```python
from build123d import *

# Parameters (mm, degrees)
PAD003_DEPTH         = 42
SKETCH008_W          = 60
SKETCH008_H          = 34
POCKET004_DEPTH      = 15.001
SKETCH009_R          = 1.45
POCKET005_DEPTH      = 8
POCKET006_DEPTH      = 42.001
POCKET008_DEPTH      = 21.001
POCKET008_DEPTH_BACK = 21.001
SKETCH013_R          = 1.75
PAD004_DEPTH         = 4.5
POCKET_DEPTH         = 25.501
PAD015_DEPTH         = 25


with BuildPart() as part:
    # Sketch006 → Pad003 (new body)
    with BuildSketch(Plane.XZ):
        with BuildLine():
            Line((-16, 21), (16, 21))
            ThreePointArc((21, 16), (19.5355339059, 19.5355339059), (16, 21))
            Line((21, 16), (21, -16))
            ThreePointArc((16, -21), (19.5355339059, -19.5355339059), (21, -16))
            Line((16, -21), (-16, -21))
            ThreePointArc((-21, -16), (-19.5355339059, -19.5355339059), (-16, -21))
            Line((-21, -16), (-21, 16))
            ThreePointArc((-16, 21), (-19.5355339059, 19.5355339059), (-21, 16))
        make_face()
    extrude(amount=PAD003_DEPTH)

    # Sketch008 (on DatumPlane) → Pocket004 (cut, through all)
    with BuildSketch(Plane.XY.offset(6)):
        with Locations((0, -17)):
            Rectangle(SKETCH008_W, SKETCH008_H)
    extrude(amount=POCKET004_DEPTH, mode=Mode.SUBTRACT)

    # Sketch009 (on DatumPlane) → Pocket005 (cut)
    with BuildSketch(Plane.XZ.offset(42)):
        with Locations((-16, 16)):
            Circle(SKETCH009_R)
        with Locations((16, 16)):
            Circle(SKETCH009_R)
        with Locations((-16, -16)):
            Circle(SKETCH009_R)
        with Locations((16, -16)):
            Circle(SKETCH009_R)
    extrude(amount=-POCKET005_DEPTH, mode=Mode.SUBTRACT)

    # Sketch010 (on DatumPlane) → Pocket006 (cut, through all)
    with BuildSketch(Plane.XZ.offset(42)):
        with BuildLine():
            Line((-18.9580398915, 15.5), (-18.9580398915, -15.5))
            ThreePointArc((-15.5, -18.9580398915), (-13.8786796564, -13.8786796564), (-18.9580398915, -15.5))
            Line((-15.5, -18.9580398915), (15.5, -18.9580398915))
            ThreePointArc((18.9580398915, -15.5), (13.8786796564, -13.8786796564), (15.5, -18.9580398915))
            Line((18.9580398915, -15.5), (18.9580398915, 15.5))
            ThreePointArc((15.5, 18.9580398915), (13.8786796564, 13.8786796564), (18.9580398915, 15.5))
            Line((-15.5, 18.9580398915), (15.5, 18.9580398915))
            ThreePointArc((-18.9580398915, 15.5), (-13.8786796564, 13.8786796564), (-15.5, 18.9580398915))
        make_face()
    extrude(amount=-POCKET006_DEPTH, mode=Mode.SUBTRACT)

    # Sketch012 → Pocket008 (cut, two sides)
    with BuildSketch(Plane.YZ) as pocket008_sk:
        with BuildLine():
            ThreePointArc((-2.5, 0), (-6, 3.5), (-9.5, 0))
            Line((-9.5, 0), (-9.5, -9))
            ThreePointArc((-9.5, -9), (-6, -12.5), (-2.5, -9))
            Line((-2.5, -9), (-2.5, 0))
        make_face()
        with BuildLine():
            ThreePointArc((-12.5, 0), (-16, 3.5), (-19.5, 0))
            Line((-19.5, 0), (-19.5, -9))
            ThreePointArc((-19.5, -9), (-16, -12.5), (-12.5, -9))
            Line((-12.5, -9), (-12.5, 0))
        make_face()
    extrude(amount=-POCKET008_DEPTH, mode=Mode.SUBTRACT)
    extrude(pocket008_sk.sketch, amount=POCKET008_DEPTH_BACK, mode=Mode.SUBTRACT)

    # Sketch013 → Pad004 (join)
    with BuildSketch(Plane.XZ):
        with BuildLine():
            ThreePointArc((22.5, 5.5), (24.9748737342, 11.4748737342), (19, 9))
            Line((19.0000000001, 9), (19.0000000001, 2.0000200959))
            ThreePointArc((22.5, 5.5), (20.0251333708, 4.4748808391), (19.0000000001, 2.0000200959))
        make_face()
        with Locations((22.5, 9)):
            Circle(SKETCH013_R, mode=Mode.SUBTRACT)
        with BuildLine():
            ThreePointArc((-22.5, -18.5), (-24.9748737342, -24.4748737342), (-19, -22))
            ThreePointArc((-18.0892857143, -19.6450903436), (-18.7643912143, -20.7375618827), (-19, -22))
            Line((-20.1450903436, -17.5892857143), (-18.0892857143, -19.6450903436))
            ThreePointArc((-22.5, -18.5), (-21.2375618827, -18.2643912143), (-20.1450903436, -17.5892857143))
        make_face()
        with Locations((-22.5, -22)):
            Circle(SKETCH013_R, mode=Mode.SUBTRACT)
        with BuildLine():
            ThreePointArc((19, -22), (24.9748737342, -24.4748737342), (22.5, -18.5))
            ThreePointArc((20.1450903436, -17.5892857143), (21.2375618827, -18.2643912143), (22.5, -18.5))
            Line((18.0892857143, -19.6450903436), (20.1450903436, -17.5892857143))
            ThreePointArc((19, -22), (18.7643912143, -20.7375618827), (18.0892857143, -19.6450903436))
        make_face()
        with Locations((22.5, -22)):
            Circle(SKETCH013_R, mode=Mode.SUBTRACT)
    extrude(amount=PAD004_DEPTH)

    # Sketch015 → Pocket (cut, through all)
    with BuildSketch(Plane.XY):
        with BuildLine():
            ThreePointArc((-12, -22), (0, -34), (12, -22))
            Line((12, -22), (12, 0))
            Line((-12, 0), (12, 0))
            Line((-12, -22), (-12, 0))
        make_face()
    extrude(amount=-POCKET_DEPTH, mode=Mode.SUBTRACT)

    # Sketch040 (on DatumPlane) → Pad015 (join)
    with BuildSketch(Plane.XY.offset(6)):
        Polygon((-19, -20), (-19, -27), (-12, -23.5), align=None)
        Polygon((19, -20), (19, -27), (12, -23.5), align=None)
    extrude(amount=-PAD015_DEPTH)


with BuildPart() as part_1:
    # Body placement: moved
    add(part.part.moved(Location((4, -6, 7))))


solid = part_1.part
```
Part model, mm, in its own coordinate system. A direction names the side the tool comes from. Coordinates: 2 decimals unless noted, no trailing zeros. Write each loop counter-clockwise with the first axis right and the second up, starting at its lowest first coordinate (ties: lowest second). Pieces come first, ordered by that corner, then holes.
Item 1: Slice it at C-C (x = 14). Write the cut outline in (y, z).
Item 2: Probe line 1 (Z direction, x = 26.5, y = -8.85); line 2 (Z direction, x = -12, y = -45); line 3 (Z direction, x = -18.5, y = -9.3). List the from-to ranges inside material, lowest first.
Item 3: Which spindle directions (+Z, -Z, +X, -X, +Y, -Y) get a long thin tool onto all of the face, cutting with end or side? Do faces 5 (the face through (-16, -22.1, -5.5)), 6 (the face through (4, -44, 25.958)), 7 (the face through (20, -40, -9)). Say none if no direction does.
Item 4: Pin check, flat tips, straight feed: pin 1 (9 mm diameter, centred on x = 8, y = -44.5, fed in from -Z); pin 2 (1 mm diameter, centred on y = -19.5, z = -13, fed in from -X); pin 3 (8 mm diameter, centred on x = 11.5, z = 22, fed in from +Y); pin 4 (4.5 mm diameter, centred on x = -18.5, z = -15, fed in from +Y). Stop position of each tip, or through.
Item 5: Slice it at A-A (y = -24). Write the cut outline in (x, z), and give its area (3 significant figures).
Item 6: Mould opens along X. For faces 1 (the face through (4, -40, -13)), 2 (the face through (-16, -12.1, -5.5)), 3 (the face through (25, -31, 4)), 4 (the face through (-13.15, -44.06, 22.12)) say: released by +X, released by -X, zero draft, split by the parting line, or undercut.
Item 7: Slice it at B-B (x = -3). Write the cut outline in (y, z).
Results found:
1. outline: (-48, -14) - (-34.63, -14) - (-34.63, -11.96) - (-48, -11.96) - close; (-48, 25.96) - (-40, 25.96) - (-40, 28) - (-48, 28) - close
2. line 1: z = -18.5 to -16.75, -13.25 to -11.5, 12.5 to 14.25, 17.75 to 19.5
2. line 2: z = -14 to -10.45, -7.55 to -6, 20 to 21.55, 24.45 to 28
2. line 3: z = -18.5 to -16.75, -13.25 to -11.5
3. face 5: +X, -X
3. face 6: +Y, -Y
3. face 7: -Y
4. pin 1: stops at z = -14
4. pin 2: stops at x = -15.57
4. pin 3: stops at y = -40
4. pin 4: stops at y = -6
5. outline: (-17, -9) arc R5 ccw to (-12, -14) - (-8, -14) - (-8, -11.96) - (-11.5, -11.96) arc R3 ccw (long way) to (-14.96, -8.5) - (-14.96, -4.87) - (-17, -4.87) - close; (-17, 9.87) - (-14.96, 9.87) - (-14.96, 13) - (-17, 13) - close; (16, -14) - (20, -14) arc R5 ccw to (25, -9) - (25, -4.87) - (22.96, -4.87) - (22.96, -8.5) arc R3 ccw (long way) to (19.5, -11.96) - (16, -11.96) - close; (22.96, 9.87) - (25, 9.87) - (25, 13) - (22.96, 13) - close
5. area: 128 mm2
6. face 1: undercut
6. face 2: zero draft
6. face 3: released by +X
6. face 4: undercut
7. outline: (-48, -14) - (-37.75, -14) - (-37.75, -11.96) - (-48, -11.96) - close; (-48, 25.96) - (-40, 25.96) - (-40, 28) - (-48, 28) - close
